Geometry: final body of the model. Coordinates: model frame, mm. A direction names the side the tool comes from. Give positions to 0.01 mm unless a question says otherwise; leave off trailing zeros. Loops run counter-clockwise (first coordinate to the right, second up) from the corner with the lowest first, then second, coordinate; pieces in that order, holes last. Notation, with made-up numbers: M 68.25,24.5 L 88.25,24.5 A18 cw 88.25,51.5 Z; hole C 80,33 d9. An arc over 180 degrees is marked long. Put each result on its own line as item: value.
```python
from build123d import *

# Parameters (mm, degrees)
SKETCH1_W               = 22.054431489
SKETCH1_H               = 12.5
BOSS_EXTRUDE1_DEPTH     = 34
CUT_EXTRUDE1_DEPTH      = 10
CUT_EXTRUDE1_DEPTH_BACK = 15
SKETCH2_R               = 1.5
FILLET3_R               = 2
SKETCH5_R               = 1.5
CUT_EXTRUDE4_DEPTH      = 52.610795679
SKETCH16_W              = 22.05443149
SKETCH16_H              = 2
CUT_EXTRUDE6_DEPTH      = 14.5
FILLET4_R               = 1


with BuildPart() as part:
    # Sketch1 → Boss-Extrude1 (new body)
    with BuildSketch(Plane.XY):
        with Locations((-13.228930986, -24.070183414)):
            Rectangle(SKETCH1_W, SKETCH1_H)
    extrude(amount=BOSS_EXTRUDE1_DEPTH)

    # Sketch2 → Cut-Extrude1 (cut, two sides: drawn at the far end of the back side and taken through both)
    with BuildSketch(Plane.XZ.offset(30.320183414).offset(-CUT_EXTRUDE1_DEPTH_BACK)):
        with Locations(Location((-13.228930986, 6.5, 0), (0, 0, 90))):
            Circle(SKETCH2_R)
        with Locations(Location((-13.228930986, 29, 0), (0, 0, 90))):
            Circle(SKETCH2_R)
        with BuildLine():
            Line((-4.315096089, 25.086165103), (-2.201715242, 25.086165103))
            add(Edge.make_bspline(
                [(-24.256146731, 25.458595261), (-35.656041951, 36.540332573), (-13.006901701, 52.285060009), (9.32231541, 36.338450422), (-2.201715242, 25.086165103)],
                knots=[0, 0, 0, 0, 0.496841919, 1, 1, 1, 1], degree=3))
            add(Edge.make_bspline(
                [(-13.228930986, 34), (-19.086447972, 37.422293362), (-24.885707195, 30.868976401), (-24.256146731, 25.458595261)],
                knots=[0, 0, 0, 0, 1, 1, 1, 1], degree=3))
            ThreePointArc((-13.228930986, 34), (-6.925897884, 31.389198205), (-4.315096089, 25.086165103))
        make_face()
        with BuildLine():
            Line((-4.478930986, 8.75), (-2.201715242, 8.75))
            add(Edge.make_bspline(
                [(-2.201715242, 8.75), (5.39210746, 3.880294823), (-0.777052631, -4.523329032), (-17.174300591, -10.623347238), (-34.821400648, -0.026005424), (-24.256146731, 8.75)],
                knots=[0, 0, 0, 0, 0.283272691, 0.504244858, 1, 1, 1, 1], degree=3))
            add(Edge.make_bspline(
                [(-23.490579314, 0), (-24.966512963, 4.237786421), (-24.256146731, 8.75)],
                knots=[0, 0, 0, 1, 1, 1], degree=2))
            Line((-23.490579314, 0), (-13.228930986, 0))
            ThreePointArc((-13.228930986, 0), (-7.041746651, 2.562815665), (-4.478930986, 8.75))
        make_face()
    extrude(amount=CUT_EXTRUDE1_DEPTH + CUT_EXTRUDE1_DEPTH_BACK, mode=Mode.SUBTRACT)

    # Fillet3
    # the kernel refuses this fillet: 2 mm, written as the material it takes off along each edge
    with BuildSketch(Plane(origin=(-24.256146731, -17.820183414, -1.998495188), x_dir=(1, 0, 0), z_dir=(0, 0, 1))) as fillet3_piece_1:
        with BuildLine():
            CenterArc((FILLET3_R, -FILLET3_R), FILLET3_R, 90, 90)
            Line((0, -FILLET3_R), (0, 0))
            Line((0, 0), (FILLET3_R, 0))
        make_face()
    extrude(amount=34.125242274, mode=Mode.SUBTRACT)
    with BuildSketch(Plane(origin=(-24.256146731, -30.320183414, -1.998495188), x_dir=(1, 0, 0), z_dir=(0, 0, 1))) as fillet3_piece_2:
        with BuildLine():
            CenterArc((FILLET3_R, FILLET3_R), FILLET3_R, 180, 90)
            Line((0, FILLET3_R), (0, 0))
            Line((0, 0), (FILLET3_R, 0))
        make_face()
    extrude(amount=34.125242274, mode=Mode.SUBTRACT)
    with BuildSketch(Plane(origin=(-24.256146731, -17.374523396, 3.001504812), x_dir=(0.1667681859257429, 1.4874647964432132e-15, -0.9859961319209304), z_dir=(0, -1, 0))) as fillet3_piece_3:
        with BuildLine():
            CenterArc((0.168096911, 1.999974157), FILLET3_R, 260.400032587, 9.891234523)
            Line((-0.165439461, 0.027981894), (0, 0))
            ThreePointArc((0, 0), (0.089132004, -0.000226606), (0.178264007, 0))
        make_face()
    extrude(amount=13.331280444, mode=Mode.SUBTRACT)
    with BuildSketch(Plane(origin=(-24.256146731, -17.482274803, 27.126747086), x_dir=(0.11756979569322837, -1.02728794699617e-15, 0.9930646218351818), z_dir=(0, -1, 0))) as fillet3_piece_4:
        with BuildLine():
            CenterArc((0.118560979, -1.999931088), FILLET3_R, 89.524368939, 7.227500304)
            Line((-0.116578613, -0.013801845), (0, 0))
            ThreePointArc((0, 0), (0.067581725, 0.000281106), (0.135163444, 0))
        make_face()
    extrude(amount=13.131401648, mode=Mode.SUBTRACT)

    # Sketch5 → Cut-Extrude4 (cut, through all)
    with BuildSketch(Plane.XY):
        with Locations((-18.011106811, -24.070183414)):
            Circle(SKETCH5_R)
        with Locations(Location((-8.446755162, -24.070183414, 0), (0, 0, 180))):
            Circle(SKETCH5_R)
    extrude(amount=CUT_EXTRUDE4_DEPTH, mode=Mode.SUBTRACT)

    # Sketch16 → Cut-Extrude6 (cut)
    with BuildSketch(Plane.XY.offset(38)):
        with Locations((-13.228930985, -20.1809771)):
            Rectangle(SKETCH16_W, SKETCH16_H)
        with Locations((-13.228930985, -28.261916897)):
            Rectangle(SKETCH16_W, SKETCH16_H)
    extrude(amount=-CUT_EXTRUDE6_DEPTH, mode=Mode.SUBTRACT)

    # Fillet4
    fillet4_edges = [part.edges().sort_by_distance(p)[0] for p in [
        (-2.201715242, -29.791050155, 25.086165103),
    ]]
    fillet(fillet4_edges, radius=FILLET4_R)


solid = part.part
```
Item 1: Section C-C on z = 25.5. Output: boundary loops of the cut face in (x, y).
Output values:
outline: M -24.26,-27.26 L -4.32,-27.26 L -4.32,-21.18 L -24.26,-21.18 Z; M -24.15,-19.18 L -4.32,-19.18 L -4.32,-17.82 L -22.26,-17.82 A2 ccw Z; M -24.02,-29.26 A2 ccw -22.26,-30.32 L -4.32,-30.32 L -4.32,-29.26 Z; hole C -18.01,-24.07 d3; hole C -8.45,-24.07 d3
Item 2: Line query: probe 1 along Y at (x, z) = (-14, 27); probe 2 along X at (y, z) = (-23.5, 18.5); probe 3 along Y at (x, z) = (-19, 27.5). Output: solid intervals per line, ascending. Write a range as [from, to].
Output values:
probe 1: [-30.32, -29.26], [-27.26, -21.18], [-19.18, -17.82]
probe 2: [-24.26, -19.4], [-16.62, -9.83], [-7.06, -2.2]
probe 3: [-30.32, -29.26], [-27.26, -25.2], [-22.94, -21.18], [-19.18, -17.82]
Item 3: Mould query, pull axis Y, two halves, no side actions, for faces 4 (the flat face through (-16, -24, 34)), 5 (the cylindrical face through (-23.686, -29.719, 15.72)), 6 (the flat face through (-16, -21.181, 29)). Classes: pulls with the +Y half, pulls with the -Y half, needs draft (parallel to the pull), parting line crosses it, or undercut.
Output values:
face 4: needs draft
face 5: pulls with the -Y half
face 6: undercut
Item 4: Pin query (flat end, axial travel): pin 1 Ø0.6 at (x, y) = (-3, -24) entering from +Z; pin 2 Ø2.5 at (x, y) = (-8.45, -24.07) entering from +Z; pin 3 Ø0.7 at (x, y) = (-3, -25) entering from -Z; pin 4 Ø2 at (x, y) = (-12, -20.5) entering from +Z. Return the tip coordinate at first contact, or that it passes through.
Output values:
pin 1: z = 25.09
pin 2: through
pin 3: z = 8.75
pin 4: z = 33.99
Item 5: Set-up query: faces 1 (the flat face through (-16, -29.262, 29)), 2 (the flat face through (-3, -18, 25.086)), 3 (the cylindrical face through (-2.5, -29.8, 24.8)). Return all of +Z, -Z, +X, -X, +Y, -Y with unobstructed straight access to the full face (end or side cutting, diameter ignored); none if empty.
Output values:
face 1: +Z, +X, -X
face 2: +Z, +X, +Y, -Y
face 3: +Z, +X, -Y
Item 6: Section D-D on y = -23.5. Count the separate pieces of the cut face and the enclosed holes in it, then the cut area to 3 significant figures.
Output values:
separate pieces: 3
enclosed holes: 2
area: 472 mm²
Item 7: Section A-A on z = 6.5. Output: boundary loops of the cut face in (x, y), then the cut area to 3 significant figures.
Output values:
outline: M -24.26,-28.32 A2 ccw -22.26,-30.32 L -14.73,-30.32 L -14.73,-17.82 L -22.26,-17.82 A2 ccw -24.26,-19.82 Z; M -11.73,-30.32 L -4.77,-30.32 L -4.77,-17.82 L -11.73,-17.82 Z; hole C -18.01,-24.07 d3; hole C -8.45,-24.07 d3
area: 190 mm²
Item 8: Section B-B on x = -15.25. Output: boundary loops of the cut face in (y, z), then the cut area to 3 significant figures.
Output values:
outline: M -30.32,0 L -17.82,0 L -17.82,34 L -19.18,34 L -19.18,23.5 L -21.18,23.5 L -21.18,34 L -27.26,34 L -27.26,23.5 L -29.26,23.5 L -29.26,34 L -30.32,34 Z
area: 383 mm²
